The model under review builds one solid part; all positions refer to its coordinate system, in mm. Round coordinates to 2 decimals unless told otherwise and drop trailing zeros. Write each loop counter-clockwise with the first axis right and the second up, starting at its lowest first coordinate (ties: lowest second). Pieces come first, ordered by that corner, then holes. Notation, with made-up numbers: (66.25, -33) -> (121.25, -33) arc R20 ccw to (121.25, -14) -> close; hole circle Ø9 at (49, 37.25). An arc over 180 degrees is marked (long way). Answer as a JSON object with one key per item and string values. Group by question number.
1) We need section B-B, the plane x = 15. Write out the cut boundary in (y, z), then the cut area to 3 significant figures.
2) Insertion check: pin 1 Ø0.6 at (y, z) = (-9.5, 1) entering from +X; pin 2 Ø0.6 at (x, z) = (-6, 1) entering from +Y. Each pin has a flat end and moves straight along its axis. Give the tip position at first contact, or say it passes through.
3) We need section A-A, the plane y = -2. Write out the cut boundary in (x, z), then the cut area to 3 significant figures.
4) We need section C-C, the plane x = 1. Write out the cut boundary in (y, z).
5) To check wall thickness, follow probe 1 along X at (y, z) = (-10.25, 1.4); probe 2 along X at (y, z) = (-8.75, 1.4); probe 3 along Y at (x, z) = (28, 1.1). State the ranges of each line that lie inside material, in increasing order. Write a range as [from, to].
from build123d import *

# Parameters (mm, degrees)
RESSALTO_EXTRUS_O1_DEPTH = 2


with BuildPart() as part:
    # Esboço1 → Ressalto-extrusão1 (new body)
    with BuildSketch(Plane.XY):
        with BuildLine():
            Line((-28.5, 0), (13, 0))
            ThreePointArc((13, 0), (13.707106781, -0.292893219), (14, -1))
            Line((14, -1), (14, -4))
            ThreePointArc((14, -4), (15, -5), (16, -4))
            Line((16, -4), (16, -1))
            ThreePointArc((16, -1), (16.292893219, -0.292893219), (17, 0))
            Line((17, 0), (28.5, 0))
            Line((28.5, 0), (26.101423641, 3.426537656))
            ThreePointArc((26.101423641, 3.426537656), (26.033676885, 4.461810381), (26.920655562, 5))
            Line((26.920655562, 5), (33, 5))
            ThreePointArc((33, 5), (33.707106781, 4.707106781), (34, 4))
            Line((34, 4), (34, -3))
            ThreePointArc((34, -3), (33.707106781, -3.707106781), (33, -4))
            Line((33, -4), (29.5, -4))
            ThreePointArc((29.5, -4), (27, -6.5), (29.5, -9))
            Line((29.5, -9), (33, -9))
            ThreePointArc((33, -9), (33.707106781, -9.292893219), (34, -10))
            Line((34, -10), (34, -14))
            ThreePointArc((34, -14), (33.707106781, -14.707106781), (33, -15))
            Line((33, -15), (13, -15))
            ThreePointArc((13, -15), (12.292893219, -14.707106781), (12, -14))
            Line((12, -14), (12, -8))
            ThreePointArc((12, -8), (11, -7), (10, -8))
            Line((10, -8), (10, -14))
            ThreePointArc((10, -14), (9.707106781, -14.707106781), (9, -15))
            Line((9, -15), (-9, -15))
            ThreePointArc((-9, -15), (-9.707106781, -14.707106781), (-10, -14))
            Line((-10, -14), (-10, -8))
            ThreePointArc((-10, -8), (-11, -7), (-12, -8))
            Line((-12, -8), (-12, -14))
            ThreePointArc((-12, -14), (-12.292893219, -14.707106781), (-13, -15))
            Line((-13, -15), (-33, -15))
            ThreePointArc((-33, -15), (-33.707106781, -14.707106781), (-34, -14))
            Line((-34, -14), (-34, -10))
            ThreePointArc((-34, -10), (-33.707106781, -9.292893219), (-33, -9))
            Line((-33, -9), (-29.5, -9))
            ThreePointArc((-29.5, -9), (-27, -6.5), (-29.5, -4))
            Line((-29.5, -4), (-33, -4))
            ThreePointArc((-33, -4), (-33.707106781, -3.707106781), (-34, -3))
            Line((-34, -3), (-34, 4))
            ThreePointArc((-34, 4), (-33.707106781, 4.707106781), (-33, 5))
            Line((-33, 5), (-26.920655562, 5))
            ThreePointArc((-26.920655562, 5), (-26.033676885, 4.461810381), (-26.101423641, 3.426537656))
            Line((-26.101423641, 3.426537656), (-28.5, 0))
        make_face()
    extrude(amount=RESSALTO_EXTRUS_O1_DEPTH)


solid = part.part
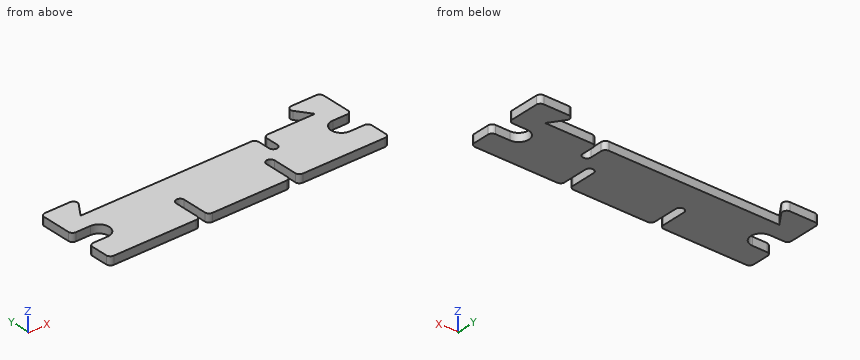
Here are the results:
{
 "1": {"outline": "(-15, 0) -> (-5, 0) -> (-5, 2) -> (-15, 2) -> close", "area": "20.0 mm^2"},
 "2": {"pin 1": "stops at x = 33.98", "pin 2": "stops at y = 0"},
 "3": {"outline": "(-34, 0) -> (14, 0) -> (14, 2) -> (-34, 2) -> close; (16, 0) -> (34, 0) -> (34, 2) -> (16, 2) -> close", "area": "132 mm^2"},
 "4": {"outline": "(-15, 0) -> (0, 0) -> (0, 2) -> (-15, 2) -> close"},
 "5": {"probe 1": "x = [-34, -12], [-10, 10], [12, 34]", "probe 2": "x = [-28.41, -12], [-10, 10], [12, 28.41]", "probe 3": "y = [-15, -8.5], [-4.5, 0], [0.71, 5]"}
}
